Can you work these out from the model? Positions are in its coordinate system, mm. Round coordinates to 2 decimals unless told otherwise and drop trailing zeros. Loops run counter-clockwise (first coordinate to the right, second up) from the corner with the lowest first, then second, coordinate; pieces in that order, holes last. Notation, with made-up numbers: (46, 76.25) -> (52, 76.25) arc R22 ccw to (52, 114.25) -> close; hole circle Ø6 at (32, -7.5). An arc over 180 degrees is marked (long way). Write each question's results on one line, items separated by ' | '.
from build123d import *

# Parameters (mm, degrees)
SKETCH1_R           = 65
BOSS_EXTRUDE1_DEPTH = 2.5
SKETCH2_R           = 13.3
CUT_EXTRUDE1_DEPTH  = 92.957870789
SKETCH3_R           = 2
CUT_EXTRUDE2_DEPTH  = 92.957870789


with BuildPart() as part:
    # Sketch1 → Boss-Extrude1 (new body)
    with BuildSketch(Plane(origin=(0, 0, 0), x_dir=(1, 0, 0), z_dir=(0, 1, 0))):
        with Locations(Location((0, 0, 0), (0, 0, 270))):
            Circle(SKETCH1_R)
    extrude(amount=BOSS_EXTRUDE1_DEPTH)

    # Sketch2 → Cut-Extrude1 (cut, through all)
    with BuildSketch(Plane.XZ):
        with Locations(Location((0, 0, 0), (0, 0, 270))):
            Circle(SKETCH2_R)
    extrude(amount=-CUT_EXTRUDE1_DEPTH, mode=Mode.SUBTRACT)

    # Sketch3 → Cut-Extrude2 (cut, through all)
    with BuildSketch(Plane.XZ):
        with Locations(Location((-41, 41, 0), (0, 0, 270))):
            Circle(SKETCH3_R)
        with Locations(Location((41, 41, 0), (0, 0, 270))):
            Circle(SKETCH3_R)
        with Locations(Location((41, -41, 0), (0, 0, 270))):
            Circle(SKETCH3_R)
        with Locations(Location((-41, -41, 0), (0, 0, 270))):
            Circle(SKETCH3_R)
    extrude(amount=-CUT_EXTRUDE2_DEPTH, mode=Mode.SUBTRACT)


solid = part.part
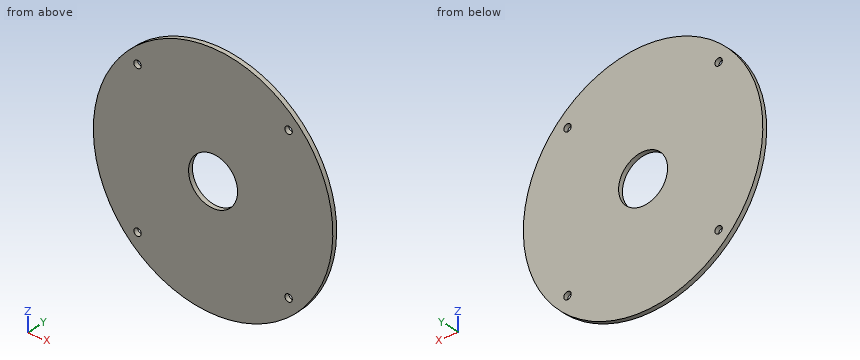
1. Please list where these lines run through material, in increasing order: line 1 (X direction, y = 1.65, z = 41); line 2 (X direction, y = 0.65, z = 0); line 3 (Z direction, x = 6, y = 1.15). Write a range as from..to.
Final values:
line 1: -50.44..-43, -39..39, 43..50.44 | line 2: -65..-13.3, 13.3..65 | line 3: -64.72..-11.87, 11.87..64.72
2. If we section it at D-D (z = -41): List the corners of the cut face in (x, y) for me.
Final values:
outline: (-50.44, 0) -> (-43, 0) -> (-43, 2.5) -> (-50.44, 2.5) -> close; (-39, 0) -> (39, 0) -> (39, 2.5) -> (-39, 2.5) -> close; (43, 0) -> (50.44, 0) -> (50.44, 2.5) -> (43, 2.5) -> close
3. If we section it at B-B (z = 0): List the corners of the cut face in (x, y) for me, then the cut area to 4 significant figures.
Final values:
outline: (-65, 0) -> (-13.3, 0) -> (-13.3, 2.5) -> (-65, 2.5) -> close; (13.3, 0) -> (65, 0) -> (65, 2.5) -> (13.3, 2.5) -> close | area: 258.5 mm2
4. If we section it at C-C (y = 0.45): List the corners of the cut face in (x, z) for me, then the cut area to 3 significant figures.
Final values:
outline: circle Ø130 at (0, 0); hole circle Ø4 at (-41, -41); hole circle Ø4 at (-41, 41); hole circle Ø26.6 at (0, 0); hole circle Ø4 at (41, -41); hole circle Ø4 at (41, 41) | area: 12,700 mm2
5. Will these pins go through, and if not, where does the flat tip stop? pin 1 (1.5 mm diameter, centred on y = 2, z = -29.5, fed in from -X); pin 2 (3 mm diameter, centred on x = -41, z = -41, fed in from +Y).
Final values:
pin 1: x = -58.3 | pin 2: through
6. If we section it at A-A (x = 0): List the corners of the cut face in (y, z) for me, then the cut area to 4 significant figures.
Final values:
outline: (0, -65) -> (2.5, -65) -> (2.5, -13.3) -> (0, -13.3) -> close; (0, 13.3) -> (2.5, 13.3) -> (2.5, 65) -> (0, 65) -> close | area: 258.5 mm2
